Geometry: see drawing. Coordinates: mm, zero at the bounding-box minimum. Round coordinates to 2 decimals unless told otherwise and drop trailing zeros. Order: outer loops, then holes, each group sorted by start corner. A loop starts at its lowest first (then second) coordinate and runs counter-clockwise, first axis right, second up. Notation, with made-up numbers: (-23, -37) -> (-13, -37) arc R15 ccw to (-13, -33) -> close; hole circle Ø4 at (14, -1.75). An arc over 180 degrees is marked (long way). One line per item, written item: value. Start each with the question number.
1) Section B-B (z = 28.1). Return the cut outline in (x, y).
2) Ray query, L1, parallel to Z at x = 28.1, y = 0.55; L2, parallel to Z at x = 29, y = 0.3. Return the intervals inside material, ascending.
3) Section C-C (y = 0.4). Return the cut outline in (x, z) (1 decimal), and give its area (3 significant figures).
4) Section A-A (x = 28.1). Return the cut outline in (y, z).
5) Pin query (flat end, axial travel): P1, Ø0.5, axis at x = 4.5, y = 0.5, coming from the +Z side; P2, Ø2, axis at x = 28.1, z = 2.8, coming from the -Y side; P3, Ø0.5, axis at x = 4, y = 0.5, coming from the -Z side. Return the tip coordinate at first contact, or that it passes through.
6) Section D-D (z = 39). Return the cut outline in (x, y).
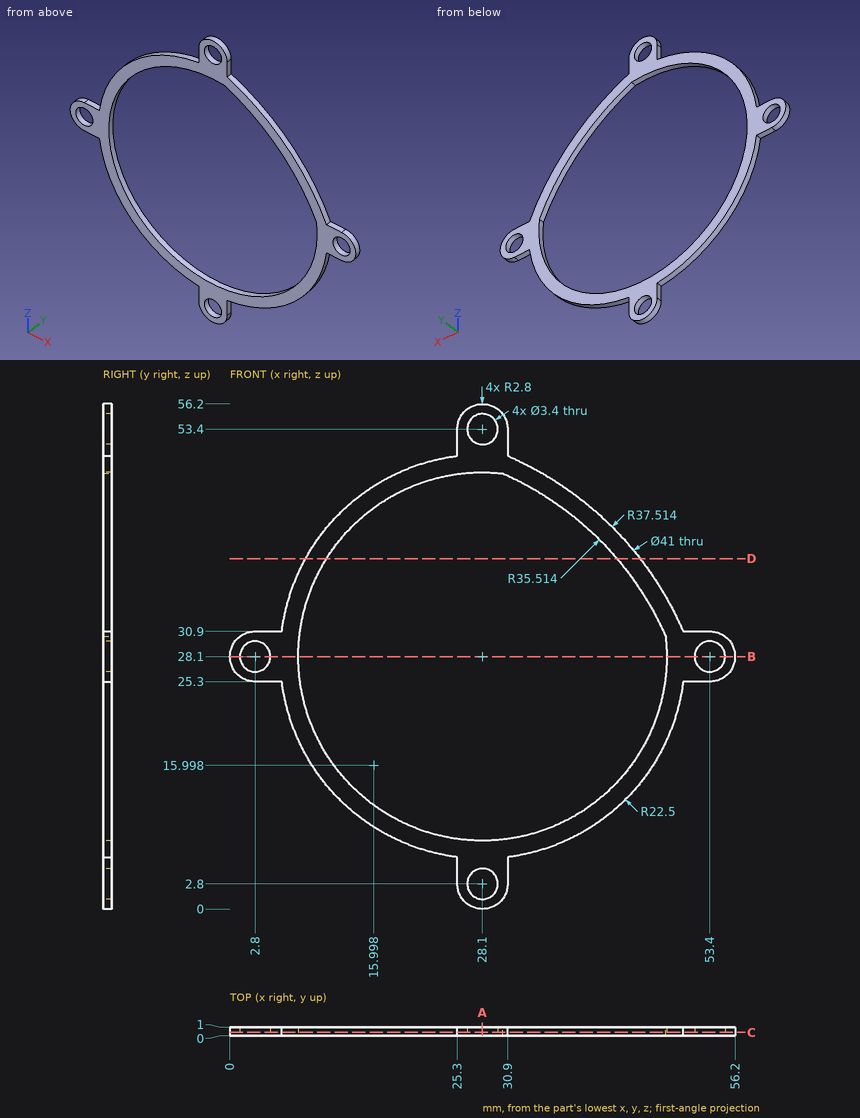
Findings:
1. outline: (0, 0) -> (1.1, 0) -> (1.1, 1) -> (0, 1) -> close; (4.5, 0) -> (7.6, 0) -> (7.6, 1) -> (4.5, 1) -> close; (48.6, 0) -> (51.7, 0) -> (51.7, 1) -> (48.6, 1) -> close; (55.1, 0) -> (56.2, 0) -> (56.2, 1) -> (55.1, 1) -> close
2. L1: 0 to 1.1, 4.5 to 7.6, 48.6 to 51.7, 55.1 to 56.2
2. L2: 0.15 to 1.36, 4.24 to 7.62, 48.58 to 51.96, 54.84 to 56.05
3. outline: (2.8, 25.3) -> (5.8, 25.3) arc R22.5 ccw to (25.3, 5.8) -> (25.3, 2.8) arc R2.8 ccw to (30.9, 2.8) -> (30.9, 5.8) arc R22.5 ccw to (50.4, 25.3) -> (53.4, 25.3) arc R2.8 ccw to (53.4, 30.9) -> (50.4, 30.9) arc R37.5 ccw to (30.9, 50.4) -> (30.9, 53.4) arc R2.8 ccw to (25.3, 53.4) -> (25.3, 50.4) arc R22.5 ccw to (5.8, 30.9) -> (2.8, 30.9) arc R2.8 ccw to start; hole circle Ø3.4 at (2.8, 28.1); hole circle Ø3.4 at (28.1, 2.8); hole circle Ø3.4 at (28.1, 53.4); hole (30.4, 48.5) arc R20.5 ccw (long way) to (48.5, 30.4) arc R35.5 ccw to start; hole circle Ø3.4 at (53.4, 28.1)
3. area: 344 mm2
4. outline: (0, 0) -> (1, 0) -> (1, 1.1) -> (0, 1.1) -> close; (0, 4.5) -> (1, 4.5) -> (1, 7.6) -> (0, 7.6) -> close; (0, 48.6) -> (1, 48.6) -> (1, 51.7) -> (0, 51.7) -> close; (0, 55.1) -> (1, 55.1) -> (1, 56.2) -> (0, 56.2) -> close
5. P1: z = 30.9
5. P2: through
5. P3: z = 25.3
6. outline: (8.42, 0) -> (10.74, 0) -> (10.74, 1) -> (8.42, 1) -> close; (43.06, 0) -> (45.63, 0) -> (45.63, 1) -> (43.06, 1) -> close
